Source: CAD feature listing. Evaluate the final solid. Frame: model axes, mm. Face numbers are marked on the shaded views. A direction names the side the tool comes from. Round coordinates to 2 decimals unless told otherwise and drop trailing zeros. Loops run counter-clockwise (first coordinate to the right, second up) from the corner with the lowest first, then second, coordinate; pieces in that order, holes last. Notation, with made-up numbers: M 79,34.5 L 132,34.5 A23 cw 132,55.5 Z; hole C 17.5,50 d10. An arc over 180 degrees is marked long. Answer as a JSON object with one key per item and string values.
from build123d import *

# Parameters (mm, degrees)
SKETCH2_W           = 13
SKETCH2_H           = 20
BOSS_EXTRUDE1_DEPTH = 6
BOSS_EXTRUDE2_DEPTH = 2
BOSS_EXTRUDE3_START = 1
SKETCH3_W           = 13
SKETCH3_H           = 20
SKETCH3_R           = 3.2
BOSS_EXTRUDE3_DEPTH = 1
BOSS_EXTRUDE4_DEPTH = 4
CUT_EXTRUDE1_START  = -6
CUT_EXTRUDE1_DEPTH  = 6
BOSS_EXTRUDE5_DEPTH = 2


# Read off the part's stored shape, not the designer's step: Cut-Extrude1
with BuildPart() as part:
    # Sketch2 → Boss-Extrude1 (new body)
    with BuildSketch(Plane.XY):
        Rectangle(SKETCH2_W, SKETCH2_H)
        with BuildLine():
            Line((1.3, -9.04), (1.3, -2.924038303))
            ThreePointArc((1.3, -2.924038303), (-3.2, 0), (1.3, 2.924038303))
            Line((1.3, 2.924038303), (1.3, 9.04))
            Line((1.3, 9.04), (5.7, 9.04))
            Line((5.7, 9.04), (5.7, -9.04))
            Line((5.7, -9.04), (1.3, -9.04))
        make_face(mode=Mode.SUBTRACT)
    extrude(amount=BOSS_EXTRUDE1_DEPTH)

    # Sketch2<3> → Boss-Extrude2 (add)
    with BuildSketch(Plane.XY):
        with BuildLine():
            Line((4.2, 7.54), (4.2, -7.54))
            Line((4.2, -7.54), (2.8, -7.54))
            Line((2.8, -7.54), (2.8, -1.549193338))
            ThreePointArc((2.8, -1.549193338), (2.162186317, -2.359014695), (1.3, -2.924038303))
            Line((1.3, -2.924038303), (1.3, -9.04))
            Line((1.3, -9.04), (5.7, -9.04))
            Line((5.7, -9.04), (5.7, 9.04))
            Line((5.7, 9.04), (1.3, 9.04))
            Line((1.3, 9.04), (1.3, 2.924038303))
            ThreePointArc((1.3, 2.924038303), (2.162186317, 2.359014695), (2.8, 1.549193338))
            Line((2.8, 1.549193338), (2.8, 7.54))
            Line((2.8, 7.54), (4.2, 7.54))
        make_face()
    extrude(amount=BOSS_EXTRUDE2_DEPTH)

    # Sketch3 → Boss-Extrude3 (add)
    with BuildSketch(Plane(origin=(0, 0, 0), x_dir=(-1, 0, 0), z_dir=(0, 0, -1)).offset(BOSS_EXTRUDE3_START)):
        Rectangle(SKETCH3_W, SKETCH3_H)
        Circle(SKETCH3_R, mode=Mode.SUBTRACT)
    extrude(amount=-BOSS_EXTRUDE3_DEPTH)

    # Sketch4 → Boss-Extrude4 (add)
    with BuildSketch(Plane.XY.offset(2)):
        with BuildLine():
            Line((2.8, 1.549193338), (2.8, 7.54))
            Line((2.8, 7.54), (4.2, 7.54))
            Line((4.2, 7.54), (4.2, -7.54))
            Line((4.2, -7.54), (2.8, -7.54))
            Line((2.8, -7.54), (2.8, -1.549193338))
            ThreePointArc((2.8, -1.549193338), (2.162186317, -2.359014695), (1.3, -2.924038303))
            Line((1.3, -2.924038303), (1.3, -9.04))
            Line((1.3, -9.04), (5.7, -9.04))
            Line((5.7, -9.04), (5.7, 9.04))
            Line((5.7, 9.04), (1.3, 9.04))
            Line((1.3, 9.04), (1.3, 2.924038303))
            ThreePointArc((1.3, 2.924038303), (2.162186317, 2.359014695), (2.8, 1.549193338))
        make_face()
    extrude(amount=BOSS_EXTRUDE4_DEPTH)

    # Cut-Extrude1 outline → Cut-Extrude1 (cut)
    with BuildSketch(Plane.XY.offset(6).offset(CUT_EXTRUDE1_START)):
        with BuildLine():
            Line((4.35, 7.69), (2.65, 7.69))
            Line((2.65, 7.69), (2.65, 1.793739111))
            ThreePointArc((2.65, 1.793739111), (2.727741861, 1.673148033), (2.8, 1.549193338))
            Line((2.8, 1.549193338), (2.8, 7.54))
            Line((2.8, 7.54), (4.2, 7.54))
            Line((4.2, 7.54), (4.2, -7.54))
            Line((4.2, -7.54), (2.8, -7.54))
            Line((2.8, -7.54), (2.8, -1.549193338))
            ThreePointArc((2.8, -1.549193338), (2.727741861, -1.673148033), (2.65, -1.793739111))
            Line((2.65, -1.793739111), (2.65, -7.69))
            Line((2.65, -7.69), (4.35, -7.69))
            Line((4.35, -7.69), (4.35, 7.69))
        make_face()
    extrude(amount=CUT_EXTRUDE1_DEPTH, mode=Mode.SUBTRACT)

    # Sketch7 → Boss-Extrude5 (add)
    with BuildSketch(Plane.XY):
        with BuildLine():
            Line((2.65, 7.69), (2.65, 1.793739111))
            ThreePointArc((2.65, 1.793739111), (3.2, 0), (2.65, -1.793739111))
            Line((2.65, -1.793739111), (2.65, -7.69))
            Line((2.65, -7.69), (4.35, -7.69))
            Line((4.35, -7.69), (4.35, 7.69))
            Line((4.35, 7.69), (2.65, 7.69))
        make_face()
    extrude(amount=BOSS_EXTRUDE5_DEPTH)


solid = part.part
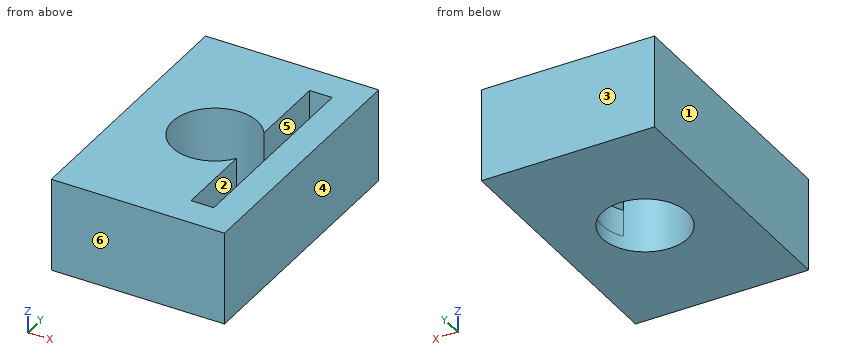
Item 1: Section B-B on y = 0. Return the cut outline in (x, z).
Answer sheet:
{"outline": "M -6.5,-1 L -3.2,-1 L -3.2,6 L -6.5,6 Z; M 3.2,-1 L 6.5,-1 L 6.5,6 L 4.35,6 L 4.35,2 L 3.2,2 Z"}
Item 2: Contact query for a flat-ended pin moving along its axis: pin 1 Ø0.8 at (x, y) = (3.5, -0.5) entering from +Z. Output: stop coordinate, or through.
Answer sheet:
{"pin 1": "stops at z = 2"}
Item 3: Line query: probe 1 along X at (y, z) = (0, 3.5); probe 2 along X at (y, z) = (0, 1.5); probe 3 along Y at (x, z) = (0, 1). Output: solid intervals per line, ascending. Write a range as from..to.
Answer sheet:
{"probe 1": "x = -6.5..-3.2, 4.35..6.5", "probe 2": "x = -6.5..-3.2, 3.2..6.5", "probe 3": "y = -10..-3.2, 3.2..10"}
Item 4: Section C-C on z = 4.25. Return the cut outline in (x, y).
Answer sheet:
{"outline": "M -6.5,-10 L 6.5,-10 L 6.5,10 L -6.5,10 Z; hole M 2.65,-7.69 L 4.35,-7.69 L 4.35,7.69 L 2.65,7.69 L 2.65,1.79 A3.2 ccw long 2.65,-1.79 Z"}
Item 5: Pull-direction query (Y, two-part tool) for the marked faces 3, 4, 5 and 6; classes: pulls with the +Y half, pulls with the -Y half, needs draft (parallel to the pull), parting line crosses it, or undercut.
Answer sheet:
{"face 3": "pulls with the +Y half", "face 4": "needs draft", "face 5": "undercut", "face 6": "pulls with the -Y half"}
Item 6: Section A-A on x = 0. Return the cut outline in (y, z).
Answer sheet:
{"outline": "M -10,-1 L -3.2,-1 L -3.2,6 L -10,6 Z; M 3.2,-1 L 10,-1 L 10,6 L 3.2,6 Z"}
Item 7: Access query for the marked faces 1 and 2. Directions: +Z, -Z, +X, -X, +Y, -Y. A direction counts if a zero-diameter tool reaches every point of the face in a straight line with its end or side. Return the directions, or none.
Answer sheet:
{"face 1": "+Z, -Z, -X, +Y, -Y", "face 2": "+Z"}
Item 8: Section D-D on x = 3.5. Return the cut outline in (y, z).
Answer sheet:
{"outline": "M -10,-1 L 10,-1 L 10,6 L 7.69,6 L 7.69,2 L -7.69,2 L -7.69,6 L -10,6 Z"}
